Can you work these out from the model? Positions are in its coordinate system, mm. Give positions to 0.01 mm unless a question says otherwise; leave off trailing zeros. Order: outer loops, then holes, each group sorted by start corner. A loop starts at its lowest first (then second) coordinate and runs counter-clockwise, first axis right, second up.
```python
from build123d import *

# Parameters (mm, degrees)
SKETCH1_W           = 13.9
SKETCH1_H           = 0.75
BOSS_EXTRUDE1_DEPTH = 0.2
SKETCH2_R           = 0.55
SKETCH2_R_2         = 3.75
CUT_EXTRUDE1_DEPTH  = 0.3
CUT_EXTRUDE2_DEPTH  = 0.3
SKETCH6_W           = 1.5
SKETCH6_H           = 1.5
BOSS_EXTRUDE2_DEPTH = 0.6
SKETCH7_W           = 0.6
SKETCH7_H           = 1.5
BOSS_EXTRUDE3_DEPTH = 1.5


with BuildPart() as part:
    # Sketch1 → Boss-Extrude1 (new body)
    with BuildSketch(Plane(origin=(0, 0, 0), x_dir=(1, 0, 0), z_dir=(0, 1, 0))):
        with BuildLine():
            Line((-13.9, 12.65), (0, 12.65))
            Line((0, 12.65), (0, 24.20560625))
            ThreePointArc((0, 24.20560625), (-0.052642553, 24.359066467), (-0.188400305, 24.447898383))
            Line((-0.188400305, 24.447898383), (-3.418729556, 25.269168531))
            ThreePointArc((-3.418729556, 25.269168531), (-3.540968219, 25.292262196), (-3.665128335, 25.3))
            Line((-3.665128335, 25.3), (-10.234871665, 25.3))
            ThreePointArc((-10.234871665, 25.3), (-10.359031781, 25.292262196), (-10.481270444, 25.269168531))
            Line((-10.481270444, 25.269168531), (-13.711599695, 24.447898383))
            ThreePointArc((-13.711599695, 24.447898383), (-13.847357447, 24.359066467), (-13.9, 24.20560625))
            Line((-13.9, 24.20560625), (-13.9, 12.65))
        make_face()
        with Locations((-6.95, 12.275)):
            Rectangle(SKETCH1_W, SKETCH1_H)
    extrude(amount=BOSS_EXTRUDE1_DEPTH)

    # Sketch2 → Cut-Extrude1 (cut)
    with BuildSketch(Plane(origin=(0, 0.2, 0), x_dir=(1, 0, 0), z_dir=(0, 1, 0))):
        with Locations((-1.11, 23.53)):
            Circle(SKETCH2_R)
        with Locations((-1.11, 12.55)):
            Circle(SKETCH2_R)
        with Locations((-12.79, 23.53)):
            Circle(SKETCH2_R)
        with Locations((-12.79, 12.55)):
            Circle(SKETCH2_R)
        with Locations((-6.95, 17.48)):
            Circle(SKETCH2_R_2)
    extrude(amount=-CUT_EXTRUDE1_DEPTH, mode=Mode.SUBTRACT)

    # Sketch4 → Cut-Extrude2 (cut)
    with BuildSketch(Plane(origin=(0, 0.2, 0), x_dir=(1, 0, 0), z_dir=(0, 1, 0))):
        with BuildLine():
            Line((-5.65, 11.9), (-8.25, 11.9))
            ThreePointArc((-8.25, 11.9), (-6.95, 13.2), (-5.65, 11.9))
        make_face()
    extrude(amount=-CUT_EXTRUDE2_DEPTH, mode=Mode.SUBTRACT)

    # Sketch6 → Boss-Extrude2 (add)
    with BuildSketch(Plane(origin=(0, 0, 0), x_dir=(0, 0, -1), z_dir=(1, 0, 0))):
        with Locations((22.05, -0.75)):
            Rectangle(SKETCH6_W, SKETCH6_H)
        with Locations((13.95, -0.75)):
            Rectangle(SKETCH6_W, SKETCH6_H)
    extrude(amount=-BOSS_EXTRUDE2_DEPTH)

    # Sketch7 → Boss-Extrude3 (add)
    with BuildSketch(Plane.XZ):
        with Locations((-0.3, -22.05)):
            Rectangle(SKETCH7_W, SKETCH7_H)
        with Locations((-0.3, -13.95)):
            Rectangle(SKETCH7_W, SKETCH7_H)
        with Locations((-13.6, -13.95)):
            Rectangle(SKETCH7_W, SKETCH7_H)
        with Locations((-13.6, -22.05)):
            Rectangle(SKETCH7_W, SKETCH7_H)
    extrude(amount=BOSS_EXTRUDE3_DEPTH)


solid = part.part
```
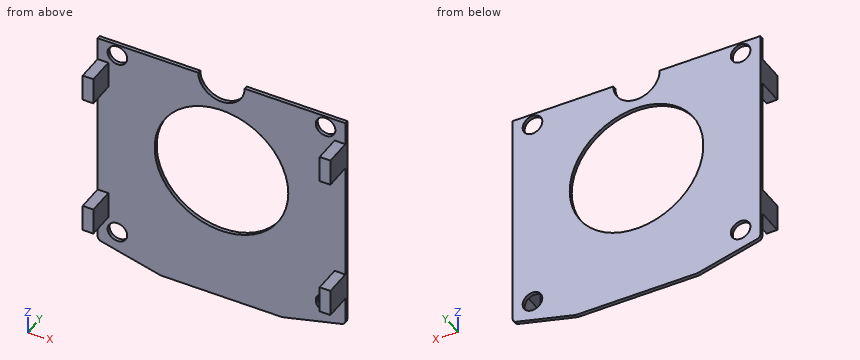
1) Suppose I cut it at B-B (z = -23.53). Please give me the cut outline in (x, y).
2) Suppose I cut it at D-D (z = -17.48). Please give me the cut outline in (x, y), and give its area (3 significant figures).
3) I'm going to push flat-ended pins straight in: pin 1 Ø5 at (x, z) = (-9.5, -13.5) entering from -Y; pin 2 Ø0.5 at (x, y) = (-13.5, -0.5) entering from +Z; pin 3 Ø1.3 at (x, z) = (-1.11, -23.53) entering from +Y. Where does each tip first touch, or does it pass through?
4) If I drill on line 1 (X direction, y = 0.15, z = -23.53); line 2 (X direction, y = -1, z = -13.5); line 3 (Z direction, x = -13.5, y = -1.05), over which ranges is the centre line in solid material (lowest first)?
5) Suppose I cut it at A-A (y = -0.45). Please give me the cut outline in (x, z), and give its area (3 significant figures).
6) Suppose I cut it at C-C (x = -6.95). Please give me the cut outline in (y, z), and give its area (3 significant figures).
Results:
1. outline: (-13.9, 0) - (-13.34, 0) - (-13.34, 0.2) - (-13.9, 0.2) - close; (-12.24, 0) - (-1.66, 0) - (-1.66, 0.2) - (-12.24, 0.2) - close; (-0.56, 0) - (0, 0) - (0, 0.2) - (-0.56, 0.2) - close
2. outline: (-13.9, 0) - (-10.7, 0) - (-10.7, 0.2) - (-13.9, 0.2) - close; (-3.2, 0) - (0, 0) - (0, 0.2) - (-3.2, 0.2) - close
2. area: 1.28 mm2
3. pin 1: stops at y = 0
3. pin 2: stops at z = -13.2
3. pin 3: stops at y = 0.2
4. line 1: x = -13.9 to -13.34, -12.24 to -1.66, -0.56 to 0
4. line 2: x = -13.9 to -13.3, -0.6 to 0
4. line 3: z = -22.8 to -21.3, -14.7 to -13.2
5. outline: (-13.9, -22.8) - (-13.3, -22.8) - (-13.3, -21.3) - (-13.9, -21.3) - close; (-13.9, -14.7) - (-13.3, -14.7) - (-13.3, -13.2) - (-13.9, -13.2) - close; (-0.6, -22.8) - (0, -22.8) - (0, -21.3) - (-0.6, -21.3) - close; (-0.6, -14.7) - (0, -14.7) - (0, -13.2) - (-0.6, -13.2) - close
5. area: 3.60 mm2
6. outline: (0, -25.3) - (0.2, -25.3) - (0.2, -21.23) - (0, -21.23) - close; (0, -13.73) - (0.2, -13.73) - (0.2, -13.2) - (0, -13.2) - close
6. area: 0.920 mm2
